```python
from build123d import *

# Parameters (mm, degrees)
F0_W      = 63.5
F0_H      = 38.1
F1_DEPTH  = 6.35
F2_W      = 44.45
F2_H      = 12.7
F3_DEPTH  = 38.1
F4_R      = 6.35
F5_DEPTH  = 25.4
F7_DEPTH  = 25.4
F10_DEPTH = 25.4
F12_DEPTH = 25.4
F13_R     = 3.175
F14_DEPTH = 25.4
F15_DEPTH = 25.4


# Not quite as in the source:
# - a feature names something its author has since deleted; it is built from what else it names


with BuildPart() as f1:
    # F0 (on Top) → F1 (new body)
    with BuildSketch(Plane.XY):
        with Locations((31.75, 19.05)):
            Rectangle(F0_W, F0_H)
    extrude(amount=F1_DEPTH)

    # F2 (on face) → F3 (join)
    with BuildSketch(Plane.XY.offset(6.35)):
        with Locations((22.225, 31.75)):
            Rectangle(F2_W, F2_H)
    extrude(amount=F3_DEPTH)

    # F4 (on face) → F5 (cut)
    with BuildSketch(Plane.XZ.offset(-25.4)):
        with Locations((12.7, 31.75)):
            Circle(F4_R)
    extrude(amount=-F5_DEPTH, mode=Mode.SUBTRACT)

    # F6 (on face) → F7 (cut)
    with BuildSketch(Plane.XZ.offset(-25.4)):
        with BuildLine():
            ThreePointArc((0, 31.7500000601), (3.7197439043, 40.7302561464), (12.7000000115, 44.45))
            Line((12.7000000115, 44.45), (0, 44.45))
            Line((0, 44.45), (0, 31.7500000601))
        make_face()
    extrude(amount=-F7_DEPTH, mode=Mode.SUBTRACT)

    # F9 (on face) → F10 (cut)
    with BuildSketch(Plane.XY.offset(6.35)):
        with BuildLine():
            ThreePointArc((6.35, 0), (2.3008253722, 2.3008253722), (0, 6.35))
            Line((0, 6.35), (0, 0))
            Line((0, 0), (6.35, 0))
        make_face()
    extrude(amount=-F10_DEPTH, mode=Mode.SUBTRACT)

    # F11 (on face) → F12 (cut)
    with BuildSketch(Plane.XY.offset(6.35)):
        with BuildLine():
            ThreePointArc((63.5, 5.8150525234), (61.7226257638, 1.7773742362), (57.6849474766, 0))
            Line((57.6849474766, 0), (63.5, 0))
            Line((63.5, 0), (63.5, 5.8150525234))
        make_face()
    extrude(amount=-F12_DEPTH, mode=Mode.SUBTRACT)

    # F13 (on face) → F14 (cut)
    with BuildSketch(Plane.XY.offset(6.35)):
        with Locations((53.975, 28.575)):
            Circle(F13_R)
        with Locations((53.975, 8.5037086033)):
            Circle(F13_R)
        with Locations((8.5037086033, 8.5037086033)):
            Circle(F13_R)
    extrude(amount=-F14_DEPTH, mode=Mode.SUBTRACT)

    # F8 (on face) → F15 (cut)
    with BuildSketch(Plane.XZ.offset(-25.4)):
        with BuildLine():
            ThreePointArc((12.7000000115, 44.45), (21.6802561251, 40.730256117), (25.4, 31.75))
            Line((25.4, 31.75), (25.4, 25.4))
            ThreePointArc((25.4, 25.4), (30.9796158184, 11.9296158184), (44.45, 6.35))
            Line((44.45, 6.35), (44.45, 44.45))
            Line((44.45, 44.45), (12.7000000115, 44.45))
        make_face()
    extrude(amount=-F15_DEPTH, mode=Mode.SUBTRACT)


solid = f1.part
```
Read the model definition and answer for the solid it produces. Units are mm, in the model's axes. A direction names the side the tool comes from. Give positions to 0.01 mm unless a question says otherwise; leave off trailing zeros. Order: outer loops, then holes, each group sorted by start corner. A loop starts at its lowest first (then second) coordinate and runs counter-clockwise, first axis right, second up. Notation, with made-up numbers: (-33.75, -11) -> (25.25, -11) arc R24 cw to (25.25, 3) -> close; hole circle Ø6 at (-33, 56.5). An arc over 180 degrees is marked (long way). Write item = value, one per line.
1. The mould has two halves that part along X. Classify faces 6 (the face through (6.356, 31.661, 32.029)), 7 (the face through (63.5, 22, 3)), 8 (the face through (50.8, 8.6, 3.2)), 9 (the face through (0, 29, 12)): +X half, -X half, draft (parallel to the pull), parting line (faces both ways), or undercut.
Numbers:
face_6 = undercut
face_7 = +X half
face_8 = undercut
face_9 = -X half
2. For faces 1 (the face through (25.4, 32, 29)), 2 (the face through (12, 25.4, 21)), 3 (the face through (31, 15, 6.35)), 4 (the face through (51.46, 26.64, 3.22)), 5 (the face through (17, 38.1, 17)), determine the directions among +Z, -Z, +X, -X, +Y, -Y from which every point of the face is accessible in a straight line to the end or side of a thin tool.
Numbers:
face_1 = +Z, +X, +Y, -Y
face_2 = +Z, +X, -X, -Y
face_3 = +Z, +X, -Y
face_4 = +Z, -Z
face_5 = +Z, -Z, +X, -X, +Y
3. Given pin 1 (10 mm diameter, centred on x = 22, y = 14.5, fed in from +Z); pin 2 (7.5 mm diameter, centred on x = 53.975, y = 28.575, fed in from +Z); pin 3 (11.5 mm diameter, centred on x = 33, y = 27.5, fed in from +Z); pin 4 (4 mm diameter, centred on x = 53.98, y = 8.5, fed in from -Z), each flat-ended and moving along its own axis, determine where each tip first touches the part or whether it passes through.
Numbers:
pin_1 = 6.35
pin_2 = 6.35
pin_3 = 17.21
pin_4 = through
4. Straight lines are drawn through the part: line 1 along Z through (x, y) = (15.5, 14); line 2 along Y through (x, z) = (13, 22); line 3 along X through (y, z) = (26, 6). For each, find the intervals that lie inside material, in ascending order.
Numbers:
line_1 = 0 to 6.35
line_2 = 25.4 to 38.1
line_3 = 0 to 52.12, 55.83 to 63.5
5. A cutting plane is placed at B-B, the plane x = 10. Write down the section's boundary in (y, z), and give its area (3 significant figures).
Numbers:
outline = (0, 0) -> (5.7, 0) -> (5.7, 6.35) -> (0, 6.35) -> close; (11.3, 0) -> (38.1, 0) -> (38.1, 26) -> (25.4, 26) -> (25.4, 6.35) -> (11.3, 6.35) -> close; (25.4, 37.5) -> (38.1, 37.5) -> (38.1, 44.16) -> (25.4, 44.16) -> close
area = 541 mm²
6. A cutting plane is placed at D-D, the plane y = 27. Write down the section's boundary in (x, z), and give its area (3 significant figures).
Numbers:
outline = (0, 0) -> (51.22, 0) -> (51.22, 6.35) -> (44.45, 6.35) arc R19.05 cw to (25.4, 25.4) -> (25.4, 31.75) arc R12.7 ccw to (0, 31.75) -> close; (56.73, 0) -> (63.5, 0) -> (63.5, 6.35) -> (56.73, 6.35) -> close; hole circle Ø12.7 at (12.7, 31.75)
area = 1,220 mm²
7. A cutting plane is placed at C-C, the plane z = 4.5. Write down the section's boundary in (x, y) (3 decimals), and give its area (3 significant figures).
Numbers:
outline = (0, 6.35) arc R8.772 ccw to (6.35, 0) -> (57.685, 0) arc R6.088 ccw to (63.5, 5.815) -> (63.5, 38.1) -> (0, 38.1) -> close; hole circle Ø6.35 at (8.504, 8.504); hole circle Ø6.35 at (53.975, 8.504); hole circle Ø6.35 at (53.975, 28.575)
area = 2,300 mm²
8. A cutting plane is placed at A-A, the plane y = 33. Write down the section's boundary in (x, z).
Numbers:
outline = (0, 0) -> (63.5, 0) -> (63.5, 6.35) -> (44.45, 6.35) arc R19.05 cw to (25.4, 25.4) -> (25.4, 31.75) arc R12.7 ccw to (0, 31.75) -> close; hole circle Ø12.7 at (12.7, 31.75)
